Study the drawing (mm; zero at the part's minimum x, y, z) and answer. Coordinates: 2 decimals unless noted, no trailing zeros. Loops run counter-clockwise (first coordinate to the right, second up) from the corner with the lowest first, then second, coordinate; pieces in that order, holes last.
Q1. Section C-C (x = 51.5) is taken. Give the vertices of the cut face in (y, z).
Q2. Section A-A (y = 49.5) is taken. Give the vertices of the cut face in (x, z), then the cut area to 3 significant figures.
Q3. A flat-ended cylindrical pin translates along its axis: P1, Ø1, axis at x = 46.5, z = 1.5, coming from the +Y side. Find the tip coordinate at first contact, or state that the pin passes through.
Q4. Section B-B (z = 0.5) is taken. Give the vertices of the cut face in (x, y).
Q5. Straight lines are drawn through the part: line 1 (X direction, y = 54, z = 0.45); line 2 (Y direction, x = 40.5, z = 0.65). For each, find the intervals that lie inside material, in ascending order.
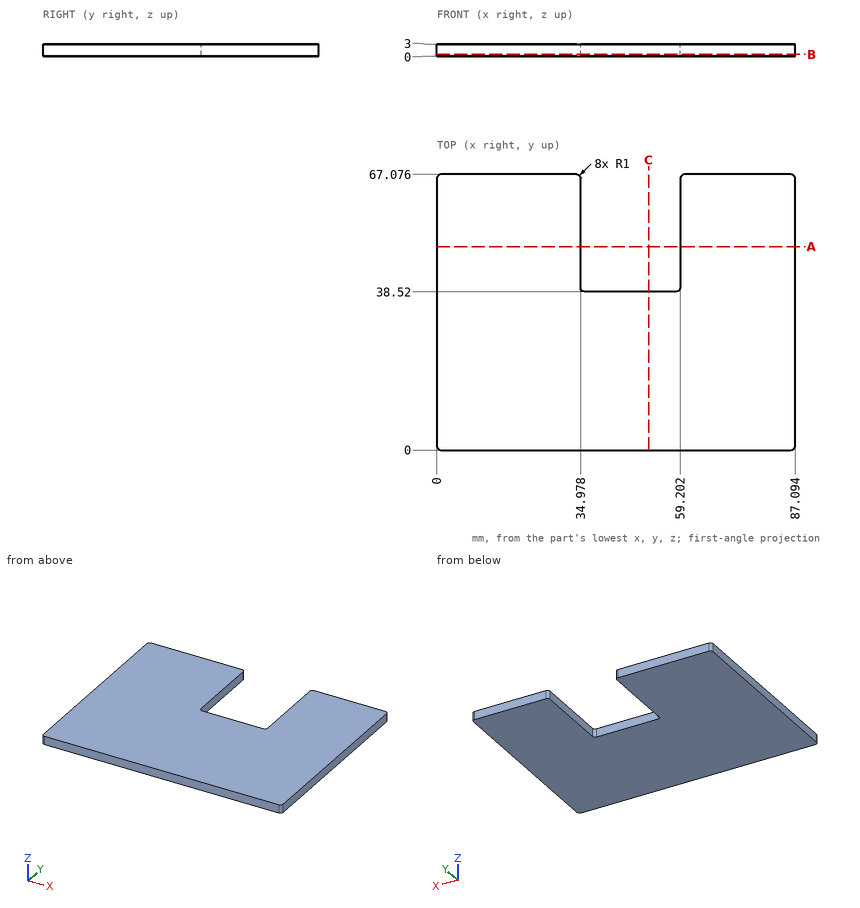
Numbers:
1. outline: (0, 0) - (38.52, 0) - (38.52, 3) - (0, 3) - close
2. outline: (0, 0) - (34.98, 0) - (34.98, 3) - (0, 3) - close; (59.2, 0) - (87.09, 0) - (87.09, 3) - (59.2, 3) - close
2. area: 189 mm2
3. P1: stops at y = 38.52
4. outline: (0, 1) arc R1 ccw to (1, 0) - (86.09, 0) arc R1 ccw to (87.09, 1) - (87.09, 66.08) arc R1 ccw to (86.09, 67.08) - (60.2, 67.08) arc R1 ccw to (59.2, 66.08) - (59.2, 39.52) arc R1 cw to (58.2, 38.52) - (35.98, 38.52) arc R1 cw to (34.98, 39.52) - (34.98, 66.08) arc R1 ccw to (33.98, 67.08) - (1, 67.08) arc R1 ccw to (0, 66.08) - close
5. line 1: x = 0 to 34.98, 59.2 to 87.09
5. line 2: y = 0 to 38.52
